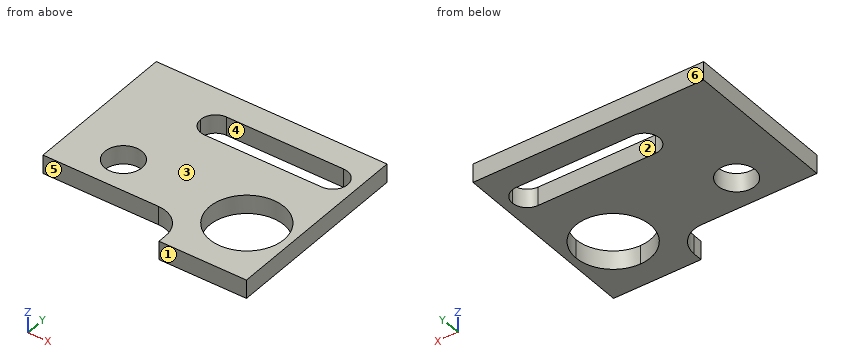
from build123d import *

# Parameters (mm, degrees)
F1_DEPTH = 25.4


with BuildPart() as f1:
    # F0 (on Top) → F1 (new body)
    with BuildSketch(Plane.XY):
        with BuildLine():
            ThreePointArc((-34.647605, -58.198605), (-60.047605, -32.798605), (-85.447605, -58.198605))
            ThreePointArc((-85.447605, -58.198605), (-60.047605, -83.598605), (-34.647605, -58.198605))
        make_face()
        with BuildLine():
            ThreePointArc((168.552395, -70.898605), (81.83137, -34.97758), (117.752395, -121.698605))
            ThreePointArc((117.752395, -121.698605), (153.673419, -106.819629), (168.552395, -70.898605))
        make_face()
        with BuildLine():
            Line((178.712395, 106.901395), (-136.247605, 106.901395))
            Line((-136.247605, 106.901395), (-136.247605, -58.198605))
            Line((-136.247605, -58.198605), (-136.247605, -103.918605))
            Line((-136.247605, -103.918605), (21.232395, -103.918605))
            ThreePointArc((21.232395, -103.918605), (48.173163, -115.077836), (59.332395, -142.018605))
            Line((59.332395, -142.018605), (59.332395, -154.718605))
            Line((59.332395, -154.718605), (117.752395, -154.718605))
            Line((117.752395, -154.718605), (178.712395, -154.718605))
            Line((178.712395, -154.718605), (178.712395, 30.701395))
            Line((178.712395, 30.701395), (178.712395, 106.901395))
        make_face()
        with BuildLine():
            ThreePointArc((-34.647605, -58.198605), (-60.047605, -83.598605), (-85.447605, -58.198605))
            ThreePointArc((-85.447605, -58.198605), (-60.047605, -32.798605), (-34.647605, -58.198605))
        make_face(mode=Mode.SUBTRACT)
        with BuildLine():
            ThreePointArc((168.552395, -70.898605), (153.673419, -106.819629), (117.752395, -121.698605))
            ThreePointArc((117.752395, -121.698605), (81.83137, -34.97758), (168.552395, -70.898605))
        make_face(mode=Mode.SUBTRACT)
        with BuildLine():
            Line((-14.327605, 71.341395), (145.692395, 71.341395))
            ThreePointArc((145.692395, 71.341395), (160.060805, 65.389805), (166.012395, 51.021395))
            ThreePointArc((166.012395, 51.021395), (160.060805, 36.652986), (145.692395, 30.701395))
            Line((145.692395, 30.701395), (-14.327605, 30.701395))
            ThreePointArc((-14.327605, 30.701395), (-28.696015, 36.652986), (-34.647605, 51.021395))
            ThreePointArc((-34.647605, 51.021395), (-28.696015, 65.389805), (-14.327605, 71.341395))
        make_face(mode=Mode.SUBTRACT)
    extrude(amount=F1_DEPTH)


solid = f1.part
The listing builds one solid part. Answer for the finished solid, in the listing's coordinates (mm). Face numbers are marked on the shaded views. A direction names the side the tool comes from. Give positions to 0.01 mm unless a question says otherwise; leave off trailing zeros. Loops run counter-clockwise (first coordinate to the right, second up) from the corner with the lowest first, then second, coordinate; pieces in that order, holes last. Notation, with made-up numbers: (11.25, -22.75) - (48.25, -22.75) arc R29 cw to (48.25, 13.25) - close; hole circle Ø9 at (39, -3.5). An arc over 180 degrees is marked (long way). Write each question's results on one line, items separated by ' | '.
1. For a pull along Y with two mould halves and no side action, classify the marked faces 1, 2 and 3 as +Y half, -Y half, draft (parallel to the pull), parting line (faces both ways), or undercut.
Resolved:
face 1: -Y half | face 2: undercut | face 3: draft
2. Flat-ended cylindrical pins translate along their axes: P1, Ø6.5, axis at y = -146, z = 19, coming from the -X side; P2, Ø7.5, axis at x = 36.5, z = 18.5, coming from the -Y side; P3, Ø1, axis at x = 17.5, z = 20.5, coming from the -Y side. Find the tip coordinate at first contact, or state that the pin passes through.
Resolved:
P1: stops at x = 59.33 | P2: stops at y = -109 | P3: stops at y = -103.92
3. Find section D-D, the plane z = 7. Write down the section's boundary in (x, y).
Resolved:
outline: (-136.25, -103.92) - (21.23, -103.92) arc R38.1 cw to (59.33, -142.02) - (59.33, -154.72) - (178.71, -154.72) - (178.71, 106.9) - (-136.25, 106.9) - close; hole circle Ø50.8 at (-60.05, -58.2); hole (-34.65, 51.02) arc R20.32 ccw to (-14.33, 30.7) - (145.69, 30.7) arc R20.32 ccw to (166.01, 51.02) arc R20.32 ccw to (145.69, 71.34) - (-14.33, 71.34) arc R20.32 ccw to start; hole (117.75, -121.7) arc R50.8 ccw to (168.55, -70.9) arc R50.8 ccw (long way) to start
4. Find section A-A, the plane x = 6.5. Write down the section's boundary in (y, z).
Resolved:
outline: (-103.92, 0) - (30.7, 0) - (30.7, 25.4) - (-103.92, 25.4) - close; (71.34, 0) - (106.9, 0) - (106.9, 25.4) - (71.34, 25.4) - close
5. Find section C-C, the plane x = 125.5. Write down the section's boundary in (y, z).
Resolved:
outline: (-154.72, 0) - (-121.1, 0) - (-121.1, 25.4) - (-154.72, 25.4) - close; (-20.69, 0) - (30.7, 0) - (30.7, 25.4) - (-20.69, 25.4) - close; (71.34, 0) - (106.9, 0) - (106.9, 25.4) - (71.34, 25.4) - close
6. Consider probe 1 along X at (y, z) = (-62.5, 9.75); probe 2 along Y at (x, z) = (131, 14); probe 3 along X at (y, z) = (-64, 7). Determine where each line is inside the solid, lowest interval first. Write a range as from..to.
Resolved:
probe 1: x = -136.25..-85.08, -35.01..67.65, 167.85..178.71 | probe 2: y = -154.72..-119.94, -21.86..30.7, 71.34..106.9 | probe 3: x = -136.25..-84.78, -35.32..67.42, 168.08..178.71
7. Which of the six approach directions +Z, -Z, +X, -X, +Y, -Y give full straight-line access (tool end or side, diameter ignored) to the marked faces 4, 5 and 6?
Resolved:
face 4: +Z, -Z | face 5: +Z, -Z, -X, -Y | face 6: +Z, -Z, +X, -X, +Y
8. Find section B-B, the plane y = 42. Write down the section's boundary in (x, z), then the cut area to 3 significant figures.
Resolved:
outline: (-136.25, 0) - (-32.54, 0) - (-32.54, 25.4) - (-136.25, 25.4) - close; (163.9, 0) - (178.71, 0) - (178.71, 25.4) - (163.9, 25.4) - close | area: 3,010 mm^2
